```python
from build123d import *

# Parameters (mm, degrees)
SKETCH1_W           = 13.6906
SKETCH1_H           = 13.6
BOSS_EXTRUDE1_DEPTH = 6.17
SKETCH2_R           = 1.651
CUT_EXTRUDE1_DEPTH  = 17.484581534
SKETCH3_W           = 6
SKETCH3_H           = 1.65
CUT_EXTRUDE2_DEPTH  = 12.452817649
SKETCH4_R           = 3.4925
CUT_EXTRUDE3_DEPTH  = 12.452817822
SKETCH5_R           = 2.54
BOSS_EXTRUDE2_DEPTH = 10.16
SKETCH6_R           = 0.889
CUT_EXTRUDE4_DEPTH  = 20.325866881


with BuildPart() as part:
    # Sketch1 → Boss-Extrude1 (new body)
    with BuildSketch(Plane.XY):
        Rectangle(SKETCH1_W, SKETCH1_H)
    extrude(amount=BOSS_EXTRUDE1_DEPTH)

    # Sketch2 → Cut-Extrude1 (cut, through all)
    with BuildSketch(Plane(origin=(6.8453, 0, 0), x_dir=(0, 0, -1), z_dir=(1, 0, 0))):
        with Locations((-2.6, 6.8)):
            Circle(SKETCH2_R)
        with Locations((-2.6, -6.8)):
            Circle(SKETCH2_R)
    extrude(amount=-CUT_EXTRUDE1_DEPTH, mode=Mode.SUBTRACT)

    # Sketch3 → Cut-Extrude2 (cut, through all)
    with BuildSketch(Plane.XY.offset(6.17)):
        with BuildLine():
            Line((-3, 5.15), (-3, 6.8))
            Line((-3, 6.8), (-4.65, 6.8))
            ThreePointArc((-4.65, 6.8), (-4.166726189, 5.633273811), (-3, 5.15))
        make_face()
        with Locations((0, 5.975)):
            Rectangle(SKETCH3_W, SKETCH3_H)
        with BuildLine():
            Line((4.65, 6.8), (3, 6.8))
            Line((3, 6.8), (3, 5.15))
            ThreePointArc((3, 5.15), (4.166726189, 5.633273811), (4.65, 6.8))
        make_face()
        with BuildLine():
            Line((3, -5.15), (3, -6.8))
            Line((3, -6.8), (4.65, -6.8))
            ThreePointArc((4.65, -6.8), (4.166726189, -5.633273811), (3, -5.15))
        make_face()
        with Locations((0, -5.975)):
            Rectangle(SKETCH3_W, SKETCH3_H)
        with BuildLine():
            Line((-4.65, -6.8), (-3, -6.8))
            Line((-3, -6.8), (-3, -5.15))
            ThreePointArc((-3, -5.15), (-4.166726189, -5.633273811), (-4.65, -6.8))
        make_face()
    extrude(amount=-CUT_EXTRUDE2_DEPTH, mode=Mode.SUBTRACT)

    # Sketch4 → Cut-Extrude3 (cut, through all)
    with BuildSketch(Plane.XY.offset(6.17)):
        Circle(SKETCH4_R)
    extrude(amount=-CUT_EXTRUDE3_DEPTH, mode=Mode.SUBTRACT)

    # Sketch5 → Boss-Extrude2 (add)
    with BuildSketch(Plane.ZY.offset(6.8453)):
        with Locations(Location((2.6, 0, 0), (0, 0, 90))):
            Circle(SKETCH5_R)
    extrude(amount=BOSS_EXTRUDE2_DEPTH)

    # Sketch6 → Cut-Extrude4 (cut, through all)
    with BuildSketch(Plane.XY.offset(6.17)):
        with Locations((-5.4356, 0)):
            Circle(SKETCH6_R)
        with Locations(Location((5.4356, 0, 0), (0, 0, 180))):
            Circle(SKETCH6_R)
    extrude(amount=-CUT_EXTRUDE4_DEPTH, mode=Mode.SUBTRACT)


solid = part.part
```
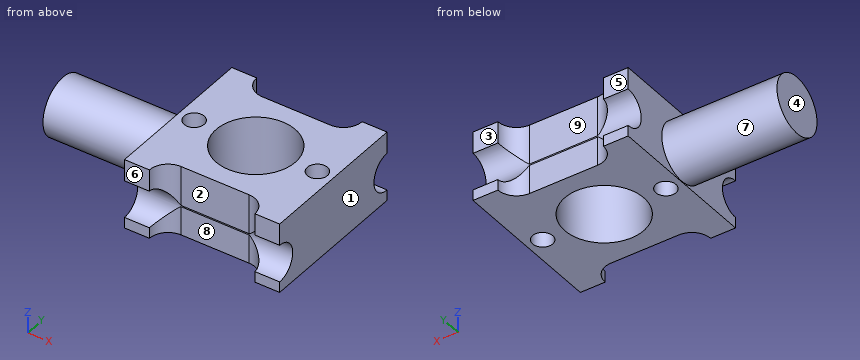
Work out the finished part from the listing and answer in its coordinate system (mm). Face numbers are marked on the shaded views. A direction names the side the tool comes from. Coordinates: 2 decimals unless noted, no trailing zeros. Write each loop counter-clockwise with the first axis right and the second up, starting at its lowest first coordinate (ties: lowest second). Pieces come first, ordered by that corner, then holes. Notation, with made-up numbers: (9.25, 72) - (57.25, 72) arc R10 ccw to (57.25, 77) - close; hole circle Ø6 at (21, 35). An arc over 180 degrees is marked (long way). Answer as a JSON object with one key per item and string values.
Q1. Find section C-C (z = 5.5). State how many separate pieces and enclosed holes the cut face has, plus the area to 3 significant figures.
Results list:
{"separate pieces": "1", "enclosed holes": "3", "area": "115 mm^2"}
Q2. Consider L1, parallel to X at y = -0.75, z = 0.75; L2, parallel to X at y = -0.5, z = 1.5; L3, parallel to Y at x = 0, z = 4.5. Determine where each line is inside the solid, lowest interval first. Write a range as from..to.
Results list:
{"L1": "x = -17.01..-5.91, -4.96..-3.41, 3.41..4.96, 5.91..6.85", "L2": "x = -17.01..-6.17, -4.7..-3.46, 3.46..4.7, 6.17..6.85", "L3": "y = -5.15..-3.49, 3.49..5.15"}
Q3. For a pull along X with two mould halves and no side action, classify the marked faces 1, 2, 3 and 4 as pulls with the +X half, pulls with the -X half, needs draft (parallel to the pull), parting line crosses it, or undercut.
Results list:
{"face 1": "pulls with the +X half", "face 2": "undercut", "face 3": "needs draft", "face 4": "pulls with the -X half"}
Q4. Find section A-A (x = 0). Write down the section's boundary in (y, z).
Results list:
{"outline": "(-5.15, 0) - (-3.49, 0) - (-3.49, 6.17) - (-5.15, 6.17) - (-5.15, 2.66) arc R1.65 cw to (-5.15, 2.54) - close; (3.49, 0) - (5.15, 0) - (5.15, 2.54) arc R1.65 cw to (5.15, 2.66) - (5.15, 6.17) - (3.49, 6.17) - close"}
Q5. Given pin 1 Ø3 at (x, z) = (2, 3.5) entering from +Y; pin 2 Ø1.8 at (x, z) = (0, 4.5) entering from -Y; pin 3 Ø2 at (x, z) = (-11, 4) entering from -Y, each flat-ended and moving along its own axis, determine where each tip first touches the part or whether it passes through.
Results list:
{"pin 1": "stops at y = 5.23", "pin 2": "stops at y = -5.15", "pin 3": "stops at y = -2.51"}
Q6. Which of the six approach directions +Z, -Z, +X, -X, +Y, -Y give full straight-line access (tool end or side, diameter ignored) to the marked faces 5, 6, 7, 8 and 9?
Results list:
{"face 5": "+Z, -Z, +X, -X, +Y", "face 6": "+Z, -Z, +X, -X, -Y", "face 7": "-X", "face 8": "+Z, -Z, -Y", "face 9": "+Z, -Z, +Y"}
Q7. Find section D-D (y = 3). Write down the section's boundary in (x, z).
Results list:
{"outline": "(-6.85, 0) - (-1.79, 0) - (-1.79, 6.17) - (-6.85, 6.17) - close; (1.79, 0) - (6.85, 0) - (6.85, 6.17) - (1.79, 6.17) - close"}
Q8. Find section B-B (y = 0). Write down the section's boundary in (x, z), plus the area to 3 significant figures.
Results list:
{"outline": "(-17.01, 0.06) - (-6.85, 0.06) - (-6.85, 0) - (-6.32, 0) - (-6.32, 6.17) - (-6.85, 6.17) - (-6.85, 5.14) - (-17.01, 5.14) - close; (-4.55, 0) - (-3.49, 0) - (-3.49, 6.17) - (-4.55, 6.17) - close; (3.49, 0) - (4.55, 0) - (4.55, 6.17) - (3.49, 6.17) - close; (6.32, 0) - (6.85, 0) - (6.85, 6.17) - (6.32, 6.17) - close", "area": "71.0 mm^2"}
